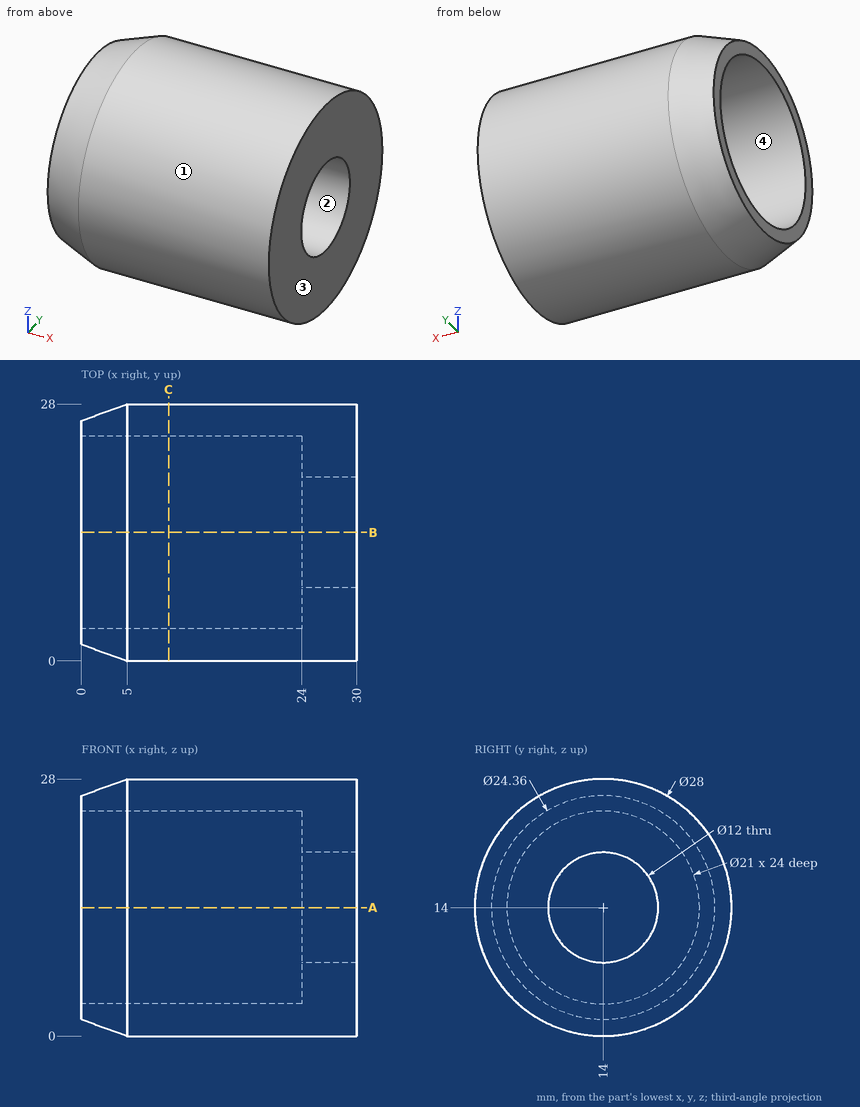
For this review, use the dimensioned drawing (mm, ordinates from the lowest corner) and the shaded views. Give positions to 0.01 mm unless a question says otherwise; leave off trailing zeros. Write each loop counter-clockwise with the first axis right and the second up, starting at its lowest first coordinate (ties: lowest second). Pieces come first, ordered by that corner, then holes. Notation, with made-up numbers: M 45,-29 L 104,-29 A21 cw 104,-5 Z; hole C 52.5,-22.5 d11. An arc over 180 degrees is marked long. Answer as a JSON object with one key per item and string values. Group by question number.
Item 1: Consider section A-A on z = 14. Write out the cut boundary in (x, y).
Item 2: For pin 1 Ø6.5 at (y, z) = (16, 12) entering from -X; pin 2 Ø1.5 at (x, z) = (26, 16) entering from -Y; pin 3 Ø2 at (x, z) = (20, 21.5) entering from +Y, all flat-tipped, find the tip position at first contact; note any pin that passes through.
Item 3: For probe 1 along Z at (x, y) = (12.25, 14); probe 2 along X at (y, z) = (21, 8.5); probe 3 along Y at (x, z) = (1.75, 19.5) (1 decimal), list the stretches that pass through material, from the lowest coordinate up. Write a range as [from, to].
Item 4: Draft analysis for pull direction Z (two halves, no side actions). For the marked faces 1, 2, 3 and 4, state which applies: +Z half, -Z half, draft (parallel to the pull), parting line (faces both ways), or undercut.
Item 5: Consider section C-C on x = 9.5. Write out the cut boundary in (y, z), plus the area to 3 significant figures.
Check result:
{
 "1": {"outline": "M 0,1.82 L 5,0 L 30,0 L 30,8 L 24,8 L 24,3.5 L 0,3.5 Z; M 0,24.5 L 24,24.5 L 24,20 L 30,20 L 30,28 L 5,28 L 0,26.18 Z"},
 "2": {"pin 1": "stops at x = 24", "pin 2": "stops at y = 0.06", "pin 3": "stops at y = 26.4"},
 "3": {"probe 1": "z = [0, 3.5], [24.5, 28]", "probe 2": "x = [24, 30]", "probe 3": "y = [2.4, 5.1], [22.9, 25.6]"},
 "4": {"face 1": "parting line", "face 2": "undercut", "face 3": "draft", "face 4": "undercut"},
 "5": {"outline": "C 14,14 d28; hole C 14,14 d21", "area": "269 mm^2"}
}
